```python
from build123d import *

# Parameters (mm, degrees)
F1_DEPTH = 10


with BuildPart() as f1:
    # F0 (on Right) → F1 (new body)
    with BuildSketch(Plane.YZ):
        Polygon((-109.380952, 198.095238), (-109.380952, -351.904762), (-9.380952, -351.904762), (-9.380952, 98.095238), (190.619048, 98.095238), (190.619048, 198.095238), align=None)
        with BuildLine():
            Line((-59.380952, -291.904762), (-59.380952, -171.904762))
            ThreePointArc((-59.380952, -171.904762), (-49.380952, -161.904762), (-39.380952, -171.904762))
            Line((-39.380952, -171.904762), (-39.380952, -291.904762))
            ThreePointArc((-39.380952, -291.904762), (-49.380952, -301.904762), (-59.380952, -291.904762))
        make_face(mode=Mode.SUBTRACT)
        with BuildLine():
            Line((-39.380952, 58.095238), (-39.380952, -61.904762))
            ThreePointArc((-39.380952, -61.904762), (-49.380952, -71.904762), (-59.380952, -61.904762))
            Line((-59.380952, -61.904762), (-59.380952, 58.095238))
            ThreePointArc((-59.380952, 58.095238), (-49.380952, 68.095238), (-39.380952, 58.095238))
        make_face(mode=Mode.SUBTRACT)
        with BuildLine():
            Line((-83.380952, 158.095238), (6.619048, 158.095238))
            ThreePointArc((6.619048, 158.095238), (16.619048, 148.095238), (6.619048, 138.095238))
            Line((6.619048, 138.095238), (-83.380952, 138.095238))
            ThreePointArc((-83.380952, 138.095238), (-93.380952, 148.095238), (-83.380952, 158.095238))
        make_face(mode=Mode.SUBTRACT)
        with BuildLine():
            Line((136.619048, 138.095238), (46.619048, 138.095238))
            ThreePointArc((46.619048, 138.095238), (36.619048, 148.095238), (46.619048, 158.095238))
            Line((46.619048, 158.095238), (136.619048, 158.095238))
            ThreePointArc((136.619048, 158.095238), (146.619048, 148.095238), (136.619048, 138.095238))
        make_face(mode=Mode.SUBTRACT)
    extrude(amount=F1_DEPTH)


solid = f1.part
```
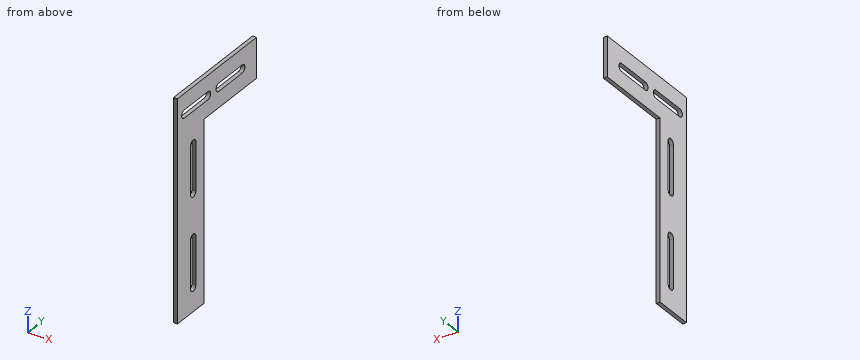
Can you work these out from the model? Positions are in its coordinate system, mm. Give positions to 0.01 mm unless a question says otherwise; leave off trailing zeros. Write each loop counter-clockwise with the first axis right and the second up, starting at its lowest first coordinate (ties: lowest second). Pieces come first, ordered by that corner, then holes. Notation, with made-up numbers: (64, 56) -> (120, 56) arc R20 ccw to (120, 73) -> close; hole circle Ø4 at (72.25, 49). An arc over 180 degrees is marked (long way). One line per item, written item: value.
Q1. Imagine slicing it at C-C on x = 7.5. Please give me the cut outline in (y, z).
Results found:
outline: (-109.38, -351.9) -> (-9.38, -351.9) -> (-9.38, 98.1) -> (190.62, 98.1) -> (190.62, 198.1) -> (-109.38, 198.1) -> close; hole (-83.38, 138.1) -> (6.62, 138.1) arc R10 ccw to (6.62, 158.1) -> (-83.38, 158.1) arc R10 ccw to start; hole (-59.38, -291.9) arc R10 ccw to (-39.38, -291.9) -> (-39.38, -171.9) arc R10 ccw to (-59.38, -171.9) -> close; hole (-59.38, -61.9) arc R10 ccw to (-39.38, -61.9) -> (-39.38, 58.1) arc R10 ccw to (-59.38, 58.1) -> close; hole (46.62, 138.1) -> (136.62, 138.1) arc R10 ccw to (136.62, 158.1) -> (46.62, 158.1) arc R10 ccw to start
Q2. Please list where these lines run through material, in increasing order: line 1 (Z direction, x = 3, y = -74); line 2 (Y direction, x = 1.75, z = 12); line 3 (Z direction, x = 1.5, y = 75). Write a range as [from, to].
Results found:
line 1: z = [-351.9, 138.1], [158.1, 198.1]
line 2: y = [-109.38, -59.38], [-39.38, -9.38]
line 3: z = [98.1, 138.1], [158.1, 198.1]
Q3. For P1, Ø3, axis at x = 3, z = -31.5, coming from the +Y side; P2, Ø3, axis at x = 7, y = 101.5, coming from the -Z side, each with a flat end and sliding along its axis, tell me the tip position at first contact or that it passes through.
Results found:
P1: stops at y = -9.38
P2: stops at z = 98.1
Q4. Imagine slicing it at D-D on z = 146. Please give me the cut outline in (x, y).
Results found:
outline: (0, -109.38) -> (10, -109.38) -> (10, -93.16) -> (0, -93.16) -> close; (0, 16.4) -> (10, 16.4) -> (10, 36.84) -> (0, 36.84) -> close; (0, 146.4) -> (10, 146.4) -> (10, 190.62) -> (0, 190.62) -> close
Q5. Imagine slicing it at A-A on y = 100. Please give me the cut outline in (x, z).
Results found:
outline: (0, 98.1) -> (10, 98.1) -> (10, 138.1) -> (0, 138.1) -> close; (0, 158.1) -> (10, 158.1) -> (10, 198.1) -> (0, 198.1) -> close
Q6. Imagine slicing it at B-B on z = -190. Please give me the cut outline in (x, y).
Results found:
outline: (0, -109.38) -> (10, -109.38) -> (10, -59.38) -> (0, -59.38) -> close; (0, -39.38) -> (10, -39.38) -> (10, -9.38) -> (0, -9.38) -> close
